Model file for the job. Use its own axes, mm. Face numbers are marked on the shaded views. Coordinates: 2 decimals unless noted, no trailing zeros. Write each loop counter-clockwise with the first axis right and the second up, starting at its lowest first coordinate (ties: lowest second). Pieces come first, ordered by that corner, then holes.
Q1. Band-saw the part on D-D, the plane z = 69. Write the cut outline in (x, y).
Q2. Band-saw the part on C-C, the plane y = 0. Write the cut outline in (x, z), plus the area to 3 significant figures.
Q3. Pull direction Z, two halves, no side cores. Call the marked faces 1, 2 and 3: released by +Z, released by -Z, zero draft, split by the parting line, or undercut.
Q4. Band-saw the part on B-B, the plane x = 31. Write the cut outline in (y, z), plus the area to 3 significant figures.
Q5. Band-saw the part on A-A, the plane y = 23. Write the cut outline in (x, z), plus the area to 3 significant figures.
Q6. Drill centre lines: probe 1 along Z at (x, y) = (-35, -4); probe 2 along Y at (x, z) = (-92, 94); probe 3 along X at (y, z) = (-3.5, 418.5). Where is each one in solid material? Low to high.
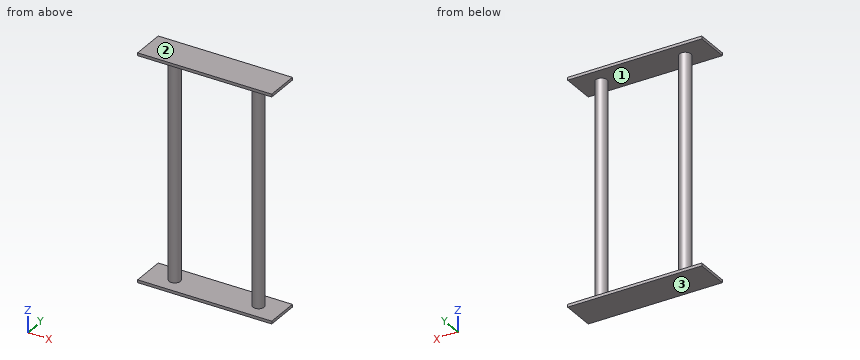
from build123d import *

# Parameters (mm, degrees)
F0_W     = 304.8
F0_H     = 76.2
F1_DEPTH = 6.35
F2_R     = 12.7
F3_DEPTH = 508
F4_W     = 304.8
F4_H     = 76.2
F4_R     = 12.7
F5_DEPTH = 6.35


with BuildPart() as f1:
    # F0 (on Top) → F1 (new body)
    with BuildSketch(Plane.XY):
        Rectangle(F0_W, F0_H)
    extrude(amount=F1_DEPTH)

    # F2 (on face) → F3 (join)
    with BuildSketch(Plane.XY.offset(6.35)):
        with Locations((-91.44, 0)):
            Circle(F2_R)
        with Locations((99.06, 0)):
            Circle(F2_R)
    extrude(amount=F3_DEPTH)

    # F4 (on face) → F5 (join)
    with BuildSketch(Plane.XY.offset(514.35)):
        Rectangle(F4_W, F4_H)
        with Locations((-91.44, 0)):
            Circle(F4_R, mode=Mode.SUBTRACT)
    extrude(amount=-F5_DEPTH)


solid = f1.part
Answer sheet:
1. outline: circle Ø25.4 at (-91.44, 0); circle Ø25.4 at (99.06, 0)
2. outline: (-152.4, 0) - (152.4, 0) - (152.4, 6.35) - (111.76, 6.35) - (111.76, 508) - (152.4, 508) - (152.4, 514.35) - (-152.4, 514.35) - (-152.4, 508) - (-104.14, 508) - (-104.14, 6.35) - (-152.4, 6.35) - close; hole (-78.74, 6.35) - (86.36, 6.35) - (86.36, 508) - (-78.74, 508) - close
2. area: 29,400 mm2
3. face 1: undercut
3. face 2: released by +Z
3. face 3: released by -Z
4. outline: (-38.1, 0) - (38.1, 0) - (38.1, 6.35) - (-38.1, 6.35) - close; (-38.1, 508) - (38.1, 508) - (38.1, 514.35) - (-38.1, 514.35) - close
4. area: 968 mm2
5. outline: (-152.4, 0) - (152.4, 0) - (152.4, 6.35) - (-152.4, 6.35) - close; (-152.4, 508) - (152.4, 508) - (152.4, 514.35) - (-152.4, 514.35) - close
5. area: 3,870 mm2
6. probe 1: z = 0 to 6.35, 508 to 514.35
6. probe 2: y = -12.69 to 12.69
6. probe 3: x = -103.65 to -79.23, 86.85 to 111.27
